Verification items for the finished model (mm, model axes). A direction names the side the tool comes from. Give positions to 0.01 mm unless a question says otherwise; leave off trailing zeros. Order: outer loops, then holes, each group sorted by start corner. A loop starts at its lowest first (then second) coordinate and runs counter-clockwise, first axis right, second up. Notation, with made-up numbers: (75.25, 78) -> (92.25, 78) arc R13 cw to (92.25, 82) -> close; hole circle Ø4 at (-31.5, -28.75). An arc over 180 degrees is marked (long way). Return JSON: item names as keys, results as strings. Group by question number.
(1) Cross-section at C-C on y = -1.35. Enter the section's corners in (x, z), then the cut area to 3 significant figures.
(2) Tool access check on faces 1 (the face through (69, -3, 21)), 2 (the face through (67, -3, 5)). Record the directions out of +Z, -Z, +X, -X, +Y, -Y that give a thin tool (end or side, any length) a straight path to the whole face; none if there is none.
(3) Cross-section at B-B on z = 5. Enter the section's corners in (x, y).
(4) Release check for a two-part mould opening along Z. For faces 3 (the face through (-1, 0, 0)), 4 (the face through (45, -3, 0)), 5 (the face through (69, -2, -21)), 6 (the face through (58.8, -3, 5)) record: pulls with the +Z half, pulls with the -Z half, needs draft (parallel to the pull), parting line crosses it, or undercut.
(5) Cross-section at A-A on x = 42.5. Enter the section's corners in (y, z), then the cut area to 3 significant figures.
(6) Thickness scan on line 1 along X through (y, z) = (-2.7, 8); line 2 along X through (y, z) = (-3.65, 19.5); line 3 along X through (y, z) = (-3.7, 19). Record the ranges inside material, lowest first.
from build123d import *

# Parameters (mm, degrees)
F0_W     = 45
F0_H     = 46
F0_W_2   = 8.2
F0_H_2   = 10
F0_W_3   = 95
F1_DEPTH = 5
F2_DEPTH = 25
F3_R     = 5


with BuildPart() as f1:
    # F0 (on Front) → F1 (new body, symmetric)
    with BuildSketch(Plane.XZ):
        with Locations((47.5, 0)):
            Rectangle(F0_W, F0_H)
        with Locations((44.7, 5)):
            Rectangle(F0_W_2, F0_H_2, mode=Mode.SUBTRACT)
        with Locations((62.9, 5)):
            Rectangle(F0_W_2, F0_H_2, mode=Mode.SUBTRACT)
        with Locations((-22.5, 0)):
            Rectangle(F0_W_3, F0_H)
    extrude(amount=F1_DEPTH, both=True)

    # F0 (on Front) → F2 (cut)
    with BuildSketch(Plane.XZ):
        with Locations((47.5, 0)):
            Rectangle(F0_W, F0_H)
        with Locations((44.7, 5)):
            Rectangle(F0_W_2, F0_H_2, mode=Mode.SUBTRACT)
        with Locations((62.9, 5)):
            Rectangle(F0_W_2, F0_H_2, mode=Mode.SUBTRACT)
        with Locations((-22.5, 0)):
            Rectangle(F0_W_3, F0_H)
    extrude(amount=-F2_DEPTH, mode=Mode.SUBTRACT)

    # F3
    f3_edges = [f1.edges().sort_by_distance(p)[0] for p in [
        (-70, -2.5, 23),
        (-70, -2.5, -23),
        (70, -2.5, 23),
        (70, -2.5, -23),
    ]]
    fillet(f3_edges, radius=F3_R)


solid = f1.part
Verdict:
{
 "1": {"outline": "(-70, -18) arc R5 ccw to (-65, -23) -> (65, -23) arc R5 ccw to (70, -18) -> (70, 18) arc R5 ccw to (65, 23) -> (-65, 23) arc R5 ccw to (-70, 18) -> close; hole (40.6, 0) -> (48.8, 0) -> (48.8, 10) -> (40.6, 10) -> close; hole (58.8, 0) -> (67, 0) -> (67, 10) -> (58.8, 10) -> close", "area": "6,250 mm²"},
 "2": {"face 1": "+Z, +X, +Y, -Y", "face 2": "+Y, -Y"},
 "3": {"outline": "(-70, -5) -> (40.6, -5) -> (40.6, 0) -> (-70, 0) -> close; (48.8, -5) -> (58.8, -5) -> (58.8, 0) -> (48.8, 0) -> close; (67, -5) -> (70, -5) -> (70, 0) -> (67, 0) -> close"},
 "4": {"face 3": "needs draft", "face 4": "undercut", "face 5": "pulls with the -Z half", "face 6": "undercut"},
 "5": {"outline": "(-5, -23) -> (0, -23) -> (0, 0) -> (-5, 0) -> close; (-5, 10) -> (0, 10) -> (0, 23) -> (-5, 23) -> close", "area": "180 mm²"},
 "6": {"line 1": "-70 to 40.6, 48.8 to 58.8, 67 to 70", "line 2": "-69.77 to 69.77", "line 3": "-69.9 to 69.9"}
}
